Read the model definition and answer for the solid it produces. Units are mm, in the model's axes. A direction names the side the tool comes from. Coordinates: 2 decimals unless noted, no trailing zeros. Loops run counter-clockwise (first coordinate to the right, second up) from the corner with the lowest first, then second, coordinate; pieces in that order, holes last. Notation, with made-up numbers: (76, 35) -> (97, 35) arc R20 ccw to (97, 51) -> close; hole circle Ø7 at (-6, -7). An arc over 180 degrees is marked (long way). Answer in a Markdown table with one row per item.
```python
from build123d import *

# Parameters (mm, degrees)
SKETCH1_W           = 25.4
SKETCH1_H           = 25.4
SKETCH1_W_2         = 22.098
SKETCH1_H_2         = 22.098
BOSS_EXTRUDE1_DEPTH = 250
SKETCH5_W           = 25.4
SKETCH5_H           = 25.4
SKETCH5_W_2         = 22.098
SKETCH5_H_2         = 22.098
BOSS_EXTRUDE2_DEPTH = 25.4
CUT_EXTRUDE1_DEPTH  = 165.021579309
CUT_EXTRUDE2_DEPTH  = 26.4


with BuildPart() as part:
    # Sketch1 → Boss-Extrude1 (new body)
    with BuildSketch(Plane.XY):
        Rectangle(SKETCH1_W, SKETCH1_H)
        Rectangle(SKETCH1_W_2, SKETCH1_H_2, mode=Mode.SUBTRACT)
    extrude(amount=-BOSS_EXTRUDE1_DEPTH)

    # Sketch5 → Boss-Extrude2 (add)
    with BuildSketch(Plane(origin=(0, 0, -250), x_dir=(-1, 0, 0), z_dir=(0, 0, -1))):
        Rectangle(SKETCH5_W, SKETCH5_H)
        Rectangle(SKETCH5_W_2, SKETCH5_H_2, mode=Mode.SUBTRACT)
    extrude(amount=BOSS_EXTRUDE2_DEPTH)

    # Sketch6 → Cut-Extrude1 (cut, through all)
    with BuildSketch(Plane(origin=(-151.321579309, -359.319373916, -111.97168159), x_dir=(0, 0, 1), z_dir=(1, 0, 0))):
        Polygon((-136.210945072, -384.704102096), (-139.845691747, -333.934645736), (-224.95481734, -363.340122949), align=None)
    extrude(amount=CUT_EXTRUDE1_DEPTH, mode=Mode.SUBTRACT)

    # Sketch7 → Cut-Extrude2 (cut, through all)
    with BuildSketch(Plane.XZ.offset(12.7)):
        Polygon((-12.7, 0), (24.645207819, -10.006618276), (24.645207819, 0), align=None)
    extrude(amount=-CUT_EXTRUDE2_DEPTH, mode=Mode.SUBTRACT)


solid = part.part
```
1. A cutting plane is placed at B-B on x = -1.75. Give the vertices of the cut face in (y, z).
A:
| item | result |
|---|---|
| outline | (-12.7, -250.91) -> (-11.05, -250.79) -> (-11.05, -2.93) -> (-12.7, -2.93) -> close; (11.05, -249.21) -> (12.7, -249.09) -> (12.7, -2.93) -> (11.05, -2.93) -> close |
2. Find the intervals of material crossed by probe 1 along Y at (x, z) = (-5.5, -141); probe 2 along Z at (x, y) = (11.75, 7), in increasing order.
A:
| item | result |
|---|---|
| probe 1 | y = -12.7 to -11.05, 11.05 to 12.7 |
| probe 2 | z = -249.5 to -6.55 |
3. A tool of negligible diameter and unlimited length cuts with its end or side. For faces 4 (the flat face through (-12.7, 0, -124)), 5 (the flat face through (0, -11.049, -124)), from which of +Z, -Z, +X, -X, +Y, -Y can it reach the whole face along a straight path? Write none if from no direction.
A:
| item | result |
|---|---|
| face 4 | +Z, -Z, -X, +Y, -Y |
| face 5 | +Z, -Z |
4. A cutting plane is placed at A-A on y = 4.75. Give the vertices of the cut face in (x, z).
A:
| item | result |
|---|---|
| outline | (-12.7, -249.66) -> (-11.05, -249.66) -> (-11.05, -0.44) -> (-12.7, 0) -> close; (11.05, -249.66) -> (12.7, -249.66) -> (12.7, -6.81) -> (11.05, -6.36) -> close |
5. A cutting plane is placed at C-C on z = -220.5. Give the vertices of the cut face in (x, y), and give its area (3 significant figures).
A:
| item | result |
|---|---|
| outline | (-12.7, -12.7) -> (12.7, -12.7) -> (12.7, 12.7) -> (-12.7, 12.7) -> close; hole (-11.05, -11.05) -> (11.05, -11.05) -> (11.05, 11.05) -> (-11.05, 11.05) -> close |
| area | 157 mm2 |
6. The mould has two halves that part along X. Classify faces 1 (the flat face through (-11.049, 0, -124)), 2 (the flat face through (12.7, 0, -127)), 3 (the flat face through (0, 12.7, -123)): pulls with the +X half, pulls with the -X half, needs draft (parallel to the pull), parting line crosses it, or undercut.
A:
| item | result |
|---|---|
| face 1 | undercut |
| face 2 | pulls with the +X half |
| face 3 | needs draft |
